Model file for the job. Use its own axes, mm. Round coordinates to 2 decimals unless told otherwise and drop trailing zeros. Loops run counter-clockwise (first coordinate to the right, second up) from the corner with the lowest first, then second, coordinate; pieces in that order, holes last. Notation, with made-up numbers: M 3.5,16 L 19.5,16 A29 ccw 19.5,48 Z; hole C 65,64.5 d5. An arc over 180 degrees is marked long. Use a Markdown table: item, result. Add a question column.
Q1. Cut at C-C (y = 4.5). Give the cut face in (x, z), plus the area to 3 significant figures.
Q2. Cut at A-A (x = -46.5). Give the cut face in (y, z), plus the area to 3 significant figures.
Q3. Mould opens along X. For faces 1 (the face through (-65, 4, 0)), 2 (the face through (-1, 0, 6)), 3 (the face through (-44.19, 4.06, -13.54)) say: +X half, -X half, draft (parallel to the pull), parting line (faces both ways), or undercut.
Q4. Pin check, flat tip, straight feed: pin 1 (3 mm diameter, centred on x = -46.5, z = -14.5, fed in from -Y). Stop position of the tip, or through.
Q5. Cut at B-B (z = 14.5). Give the cut face in (x, y), plus the area to 3 significant figures.
Q6. Cut at D-D (x = 0). Give the cut face in (y, z), plus the area to 3 significant figures.
Q7. Probe line 1 (Z direction, x = 46.5, y = 2.25); line 2 (X direction, y = 5, z = 14.5); line 3 (X direction, y = 3.75, z = 0). List the from-to ranges inside material, lowest first. Write a range as from..to.
from build123d import *

# Parameters (mm, degrees)
SKETCH_1_W          = 130
SKETCH_1_H          = 60
EXTRUDE_1_DEPTH     = 8
SKETCH_2_R          = 2.5
CUT_EXTRUDE_1_DEPTH = 9


with BuildPart() as part:
    # ｽｹｯﾁ1 → ﾎﾞｽ - 押し出し1 (new body)
    with BuildSketch(Plane(origin=(0, 0, 0), x_dir=(1, 0, 0), z_dir=(0, 1, 0))):
        Rectangle(SKETCH_1_W, SKETCH_1_H)
    extrude(amount=EXTRUDE_1_DEPTH)

    # ｽｹｯﾁ2 → ｶｯﾄ - 押し出し1 (cut, through all)
    with BuildSketch(Plane(origin=(0, 8, 0), x_dir=(1, 0, 0), z_dir=(0, 1, 0))):
        Circle(SKETCH_2_R)
        with Locations((59, 0)):
            Circle(SKETCH_2_R)
        with Locations((46.5, -14.5)):
            Circle(SKETCH_2_R)
        with Locations((46.5, 14.5)):
            Circle(SKETCH_2_R)
        with Locations((-46.5, -14.5)):
            Circle(SKETCH_2_R)
        with Locations((-59, 0)):
            Circle(SKETCH_2_R)
        with Locations((-46.5, 14.5)):
            Circle(SKETCH_2_R)
    extrude(amount=-CUT_EXTRUDE_1_DEPTH, mode=Mode.SUBTRACT)


solid = part.part
Checked values:
| question | item | result |
|---|---|---|
| 1 | outline | M -65,-30 L 65,-30 L 65,30 L -65,30 Z; hole C -59,0 d5; hole C -46.5,-14.5 d5; hole C -46.5,14.5 d5; hole C 0,0 d5; hole C 46.5,-14.5 d5; hole C 46.5,14.5 d5; hole C 59,0 d5 |
| 1 | area | 7,660 mm^2 |
| 2 | outline | M 0,-30 L 8,-30 L 8,-17 L 0,-17 Z; M 0,-12 L 8,-12 L 8,12 L 0,12 Z; M 0,17 L 8,17 L 8,30 L 0,30 Z |
| 2 | area | 400 mm^2 |
| 3 | face 1 | -X half |
| 3 | face 2 | draft |
| 3 | face 3 | undercut |
| 4 | pin 1 | passes through |
| 5 | outline | M -65,0 L -49,0 L -49,8 L -65,8 Z; M -44,0 L 44,0 L 44,8 L -44,8 Z; M 49,0 L 65,0 L 65,8 L 49,8 Z |
| 5 | area | 960 mm^2 |
| 6 | outline | M 0,-30 L 8,-30 L 8,-2.5 L 0,-2.5 Z; M 0,2.5 L 8,2.5 L 8,30 L 0,30 Z |
| 6 | area | 440 mm^2 |
| 7 | line 1 | z = -30..-17, -12..12, 17..30 |
| 7 | line 2 | x = -65..-49, -44..44, 49..65 |
| 7 | line 3 | x = -65..-61.5, -56.5..-2.5, 2.5..56.5, 61.5..65 |
